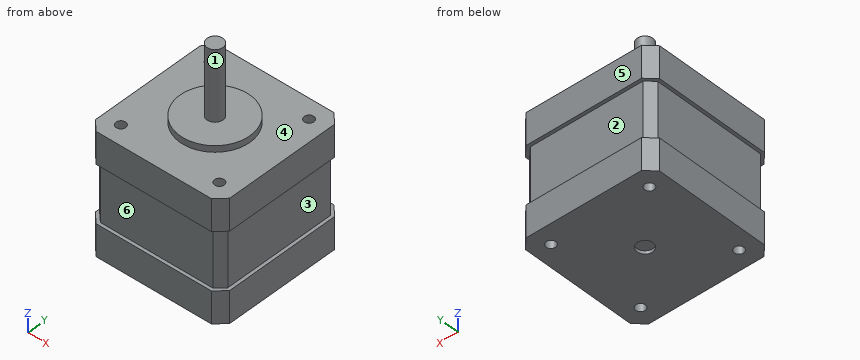
```python
from build123d import *

# Parameters (mm, degrees)
EXTRUDE_1_DEPTH     = 10
SKETCH_2_R          = 11
EXTRUDE_2_DEPTH     = 2
SKETCH_3_R          = 2.5
EXTRUDE_3_DEPTH     = 22
EXTRUDE_4_DEPTH     = 18
EXTRUDE_5_DEPTH     = 10
SKETCH_4_R          = 1.5
CUT_EXTRUDE_1_DEPTH = 46.5
SKETCH_5_R          = 2.5
CUT_EXTRUDE_2_DEPTH = 1


with BuildPart() as part:
    # Эскиз1 → Бобышка-Вытянуть1 (new body)
    with BuildSketch(Plane.XY):
        Polygon((-32.767753805, -16.536194896), (-32.767753805, 19.763805104), (-29.767753805, 22.763805104), (6.532246195, 22.763805104), (9.532246195, 19.763805104), (9.532246195, -16.536194896), (6.532246195, -19.536194896), (-29.767753805, -19.536194896), align=None)
    extrude(amount=EXTRUDE_1_DEPTH)

    # Эскиз2 → Бобышка-Вытянуть2 (add)
    with BuildSketch(Plane.XY.offset(10)):
        with Locations((-11.617753805, 1.613805104)):
            Circle(SKETCH_2_R)
    extrude(amount=EXTRUDE_2_DEPTH)

    # Эскиз3 → Бобышка-Вытянуть3 (add)
    with BuildSketch(Plane.XY.offset(12)):
        with Locations((-11.617753805, 1.613805104)):
            Circle(SKETCH_3_R)
    extrude(amount=EXTRUDE_3_DEPTH)

    # Эскиз6 → Бобышка-Вытянуть4 (add)
    with BuildSketch(Plane(origin=(0, 0, 0), x_dir=(-1, 0, 0), z_dir=(0, 0, -1))):
        Polygon((11.617753805, 21.763805104), (-6.118032632, 21.763805104), (-8.532246195, 19.349591542), (-8.532246195, -16.121981333), (-6.118032632, -18.536194896), (29.353540243, -18.536194896), (31.767753805, -16.121981333), (31.767753805, 19.349591542), (29.353540243, 21.763805104), align=None)
    extrude(amount=EXTRUDE_4_DEPTH)

    # Эскиз7 → Бобышка-Вытянуть5 (add)
    with BuildSketch(Plane.XY.offset(-18)):
        Polygon((-32.767753805, -16.536194896), (-32.767753805, 19.763805104), (-29.767753805, 22.763805104), (6.532246195, 22.763805104), (9.532246195, 19.763805104), (9.532246195, -16.536194896), (6.532246195, -19.536194896), (-29.767753805, -19.536194896), align=None)
    extrude(amount=-EXTRUDE_5_DEPTH)

    # Эскиз4 → Вырез-Вытянуть1 (cut)
    with BuildSketch(Plane.XY.offset(10)):
        with Locations((-27.117753805, 17.113805104)):
            Circle(SKETCH_4_R)
        with Locations((3.882246195, 17.113805104)):
            Circle(SKETCH_4_R)
        with Locations((3.882246195, -13.886194896)):
            Circle(SKETCH_4_R)
        with Locations((-27.117753805, -13.886194896)):
            Circle(SKETCH_4_R)
    extrude(amount=-CUT_EXTRUDE_1_DEPTH, mode=Mode.SUBTRACT)

    # Эскиз5 → Вырез-Вытянуть2 (cut)
    with BuildSketch(Plane(origin=(0, 0, -28), x_dir=(-1, 0, 0), z_dir=(0, 0, -1))):
        with Locations((11.617753805, 1.613805104)):
            Circle(SKETCH_5_R)
    extrude(amount=-CUT_EXTRUDE_2_DEPTH, mode=Mode.SUBTRACT)


solid = part.part
```
Check sheet for the modelled part. Datum: model origin and axes. Units: mm. Face numbers are marked on the shaded views. A direction names the side the tool comes from. Give positions to 0.01 mm unless a question says otherwise; leave off trailing zeros. Order: outer loops, then holes, each group sorted by start corner. A loop starts at its lowest first (then second) coordinate and runs counter-clockwise, first axis right, second up. Notation, with made-up numbers: (47.25, 39.5) -> (104.25, 39.5) arc R25 cw to (104.25, 77.5) -> close; hole circle Ø4 at (89.5, 78). An arc over 180 degrees is marked (long way). Use CSV: the item, a comma, the result in double quotes. Start each with the question number.
1) Sectioned sample at C-C, the plane z = 9. Record the boundary of the cut face in (x, y), plus the area to 3 significant figures.
2) Sectioned sample at A-A, the plane y = 10.5. Record the boundary of the cut face in (x, z).
3) Material ranges on line 1 (X direction, y = 18, z = -2); line 2 (Y direction, x = -28, z = -16.5); line 3 (X direction, y = 8, z = -17), recorded low to high. Write a range as from..to.
4) Go/stop test with flat-tipped pins: P1, Ø10, axis at x = -1, y = 5.5, coming from the +Z side; P2, Ø5.5, axis at x = -8.5, z = -6, coming from the +Y side; P3, Ø5.5, axis at y = 0, z = -6, coming from the +X side. Record where each tip stops, or that it passes through.
5) Mould release check, pull along Z, two halves, no side actions. Record for the marked faces 4, 5 and 6: released by +Z, released by -Z, zero draft, split by the parting line, or undercut.
6) Sectioned sample at D-D, the plane z = -6. Record the boundary of the cut face in (x, y), plus the area to 3 significant figures.
7) Sectioned sample at B-B, the plane x = -13. Record the boundary of the cut face in (y, z).
8) Set-up check for the marked faces 1, 2 and 3: record each of +Z, -Z, +X, -X, +Y, -Y from which the full face is reachable in a straight line by a thin tool's end or side.
Recorded:
1,outline,"(-32.77, -16.54) -> (-29.77, -19.54) -> (6.53, -19.54) -> (9.53, -16.54) -> (9.53, 19.76) -> (6.53, 22.76) -> (-29.77, 22.76) -> (-32.77, 19.76) -> close; hole circle Ø3 at (-27.12, -13.89); hole circle Ø3 at (-27.12, 17.11); hole circle Ø3 at (3.88, -13.89); hole circle Ø3 at (3.88, 17.11)"
1,area,"1,740 mm2"
2,outline,"(-32.77, -28) -> (9.53, -28) -> (9.53, -18) -> (8.53, -18) -> (8.53, 0) -> (9.53, 0) -> (9.53, 10) -> (-5.13, 10) -> (-5.13, 12) -> (-18.1, 12) -> (-18.1, 10) -> (-32.77, 10) -> (-32.77, 0) -> (-31.77, 0) -> (-31.77, -18) -> (-32.77, -18) -> close"
3,line 1,"-31.77..-28.33, -25.91..2.67, 5.09..8.53"
3,line 2,"-18.54..-15.1, -12.67..15.9, 18.33..21.76"
3,line 3,"-31.77..8.53"
4,P1,"z = 12"
4,P2,"y = 21.76"
4,P3,"x = 8.53"
5,face 4,"released by +Z"
5,face 5,"zero draft"
5,face 6,"undercut"
6,outline,"(-31.77, -16.12) -> (-29.35, -18.54) -> (6.12, -18.54) -> (8.53, -16.12) -> (8.53, 19.35) -> (6.12, 21.76) -> (-29.35, 21.76) -> (-31.77, 19.35) -> close; hole circle Ø3 at (-27.12, -13.89); hole circle Ø3 at (-27.12, 17.11); hole circle Ø3 at (3.88, -13.89); hole circle Ø3 at (3.88, 17.11)"
6,area,"1,580 mm2"
7,outline,"(-19.54, -28) -> (-0.47, -28) -> (-0.47, -27) -> (3.7, -27) -> (3.7, -28) -> (22.76, -28) -> (22.76, -18) -> (21.76, -18) -> (21.76, 0) -> (22.76, 0) -> (22.76, 10) -> (12.53, 10) -> (12.53, 12) -> (3.7, 12) -> (3.7, 34) -> (-0.47, 34) -> (-0.47, 12) -> (-9.3, 12) -> (-9.3, 10) -> (-19.54, 10) -> (-19.54, 0) -> (-18.54, 0) -> (-18.54, -18) -> (-19.54, -18) -> close"
8,face 1,"+Z"
8,face 2,"+X, -X, +Y"
8,face 3,"+X, +Y, -Y"
